from build123d import *

# Parameters (mm, degrees)
F0_R     = 1.625
F0_R_2   = 4
F0_R_3   = 3
F1_DEPTH = 4
F3_DEPTH = 25
F5_DEPTH = 2
F6_R     = 1


with BuildPart() as f1:
    # F0 (on Top) → F1 (new body)
    with BuildSketch(Plane.XY):
        with BuildLine():
            ThreePointArc((-9.4837298081, 16.9083510106), (-10.0814206469, 18.2972590095), (-11.0073593129, 19.4926406871))
            Line((-11.0073593129, 19.4926406871), (-39.7406588467, 48.2259402209))
            ThreePointArc((-39.7406588467, 48.2259402209), (-45.1494727757, 55.6091692733), (-48.0804471902, 64.2796207229))
            ThreePointArc((-48.0804471902, 64.2796207229), (-52.3618521384, 72.1460862496), (-60.5351583135, 75.8078855862))
            ThreePointArc((-60.5351583135, 75.8078855862), (-65.6898975166, 76.7624502228), (-70.5997654152, 78.5997654152))
            ThreePointArc((-70.5997654152, 78.5997654152), (-77.4281925399, 77.4281925399), (-78.5997654152, 70.5997654152))
            ThreePointArc((-78.5997654152, 70.5997654152), (-76.7624502228, 65.6898975166), (-75.8078855862, 60.5351583135))
            ThreePointArc((-75.8078855862, 60.5351583135), (-72.1460862496, 52.3618521384), (-64.2796207229, 48.0804471902))
            ThreePointArc((-64.2796207229, 48.0804471902), (-55.6091692733, 45.1494727757), (-48.2259402209, 39.7406588467))
            Line((-48.2259402209, 39.7406588467), (-19.4926406871, 11.0073593129))
            ThreePointArc((-19.4926406871, 11.0073593129), (-18.2972590095, 10.0814206469), (-16.9083510106, 9.4837298081))
            ThreePointArc((-16.9083510106, 9.4837298081), (-14.5935043457, 8.4875784101), (-12.6012015497, 6.9443473002))
            Line((-12.6012015497, 6.9443473002), (-5.6568542495, 0))
            Line((-5.6568542495, 0), (0, 0))
            Line((0, 0), (0, 5.6568542495))
            Line((0, 5.6568542495), (-6.9443473002, 12.6012015497))
            ThreePointArc((-6.9443473002, 12.6012015497), (-8.4875784101, 14.5935043457), (-9.4837298081, 16.9083510106))
        make_face()
        with Locations((-15.25, 15.25)):
            Circle(F0_R, mode=Mode.SUBTRACT)
        with Locations((-21, 21)):
            Circle(F0_R, mode=Mode.SUBTRACT)
        with Locations((-61.8718433538, 61.8718433538)):
            Circle(F0_R_2, mode=Mode.SUBTRACT)
        with Locations((-73.1855518528, 73.1855518528)):
            Circle(F0_R_3, mode=Mode.SUBTRACT)
    extrude(amount=F1_DEPTH)

    # F2 (on face) → F3 (cut)
    with BuildSketch(Plane.XY.offset(4)):
        with BuildLine():
            ThreePointArc((-55.3718433538, 63.4718433538), (-56.9718433538, 61.8718433538), (-55.3718433538, 60.2718433538))
            Line((-55.3718433538, 60.2718433538), (-52.3718433538, 60.2718433538))
            ThreePointArc((-52.3718433538, 60.2718433538), (-50.7718433538, 61.8718433538), (-52.3718433538, 63.4718433538))
            Line((-52.3718433538, 63.4718433538), (-55.3718433538, 63.4718433538))
        make_face()
        with BuildLine():
            Line((-63.4718433538, 71.3718433538), (-63.4718433538, 68.3718433538))
            ThreePointArc((-63.4718433538, 68.3718433538), (-61.8718433538, 66.7718433538), (-60.2718433538, 68.3718433538))
            Line((-60.2718433538, 68.3718433538), (-60.2718433538, 71.3718433538))
            ThreePointArc((-60.2718433538, 71.3718433538), (-61.8718433538, 72.9718433538), (-63.4718433538, 71.3718433538))
        make_face()
        with BuildLine():
            Line((-71.3718433538, 60.2718433538), (-68.3718433538, 60.2718433538))
            ThreePointArc((-68.3718433538, 60.2718433538), (-66.7718433538, 61.8718433538), (-68.3718433538, 63.4718433538))
            Line((-68.3718433538, 63.4718433538), (-71.3718433538, 63.4718433538))
            ThreePointArc((-71.3718433538, 63.4718433538), (-72.9718433538, 61.8718433538), (-71.3718433538, 60.2718433538))
        make_face()
        with BuildLine():
            Line((-60.2718433538, 52.3718433538), (-60.2718433538, 55.3718433538))
            ThreePointArc((-60.2718433538, 55.3718433538), (-61.8718433538, 56.9718433538), (-63.4718433538, 55.3718433538))
            Line((-63.4718433538, 55.3718433538), (-63.4718433538, 52.3718433538))
            ThreePointArc((-63.4718433538, 52.3718433538), (-61.8718433538, 50.7718433538), (-60.2718433538, 52.3718433538))
        make_face()
    extrude(amount=-F3_DEPTH, mode=Mode.SUBTRACT)

    # F4 (on face) → F5 (cut)
    with BuildSketch(Plane(origin=(0, 0, 0), x_dir=(1, 0, 0), z_dir=(0, 0, -1))):
        with BuildLine():
            Line((0, 0), (-20, 0))
            Line((-20, 0), (-20, -10.25))
            Line((-20, -10.25), (-15.25, -10.25))
            ThreePointArc((-15.25, -10.25), (-11.7144660941, -11.7144660941), (-10.25, -15.25))
            Line((-10.25, -15.25), (-10.25, -20))
            Line((-10.25, -20), (0, -20))
            Line((0, -20), (0, 0))
        make_face()
    extrude(amount=-F5_DEPTH, mode=Mode.SUBTRACT)

    # F6
    f6_edges = [f1.edges().sort_by_distance(p)[0] for p in [
        (0, 0, 3),
    ]]
    fillet(f6_edges, radius=F6_R)


solid = f1.part
Read the model definition and answer for the solid it produces. Units are mm, in the model's axes. A direction names the side the tool comes from. Coordinates: 2 decimals unless noted, no trailing zeros. Order: outer loops, then holes, each group sorted by start corner. A loop starts at its lowest first (then second) coordinate and runs counter-clockwise, first axis right, second up. Notation, with made-up numbers: M -35.75,-21.5 L -12.75,-21.5 A8 ccw -12.75,-15.5 Z; hole C 85,-2 d6. An arc over 180 degrees is marked long. Put each result on its own line as item: value. Start each with the question number.
Item 1: Section A-A, the plane x = -54 is taken. Determine the outline of the cut face in (y, z), plus the area to 3 significant figures.
Item 2: Given pin 1 Ø1.5 at (x, z) = (-54, 2.5) entering from +Y; pin 2 Ø1.5 at (y, z) = (54.5, 2.5) entering from +X; pin 3 Ø1.5 at (x, z) = (-70, 2) entering from +Y, each flat-ended and moving along its own axis, determine where each tip first touches the part or whether it passes through.
Item 3: The mould has two halves that part along X. Classify faces 1 (the face through (-9.178, 3.521, 2.986)), 2 (the face through (-45.09, 55.495, 1.972)), 3 (the face through (-54, 63.472, 2)): +X half, -X half, draft (parallel to the pull), parting line (faces both ways), or undercut.
Item 4: Section C-C, the plane y = 34 is taken. Determine the outline of the cut face in (x, z).
Item 5: For faces 4 (the face through (-10.249, 18.565, 2.416)), 5 (the face through (-10.25, 17, 1)), 6 (the face through (-72.97, 61.91, 2.03)), determine the directions among +Z, -Z, +X, -X, +Y, -Y from which every point of the face is accessible in a straight line to the end or side of a thin tool.
Item 6: Consider probe 1 along X at (y, z) = (71, 2.15); probe 2 along Y at (x, z) = (-62, 3.4); probe 3 along Z at (x, y) = (-9, 7). Determine where each line is inside the solid, lowest interval first. Write a range as [from, to].
Item 7: Section B-B, the plane y = 21 is taken. Determine the outline of the cut face in (x, z) (3 decimals), plus the area to 3 significant figures.
Computed:
1. outline: M 44.25,0 L 60.27,0 L 60.27,4 L 44.25,4 Z; M 63.47,0 L 73.45,0 L 73.45,4 L 63.47,4 Z
1. area: 104 mm2
2. pin 1: stops at y = 73.93
2. pin 2: stops at x = -44.1
2. pin 3: stops at y = 78.67
3. face 1: -X half
3. face 2: +X half
3. face 3: undercut
4. outline: M -42.49,0 L -25.51,0 L -25.51,4 L -42.49,4 Z
5. face 4: +Z, -Z, +X, +Y
5. face 5: -Z, +X, +Y, -Y
5. face 6: +Z, -Z
6. probe 1: x = [-78.77, -75.24], [-71.13, -63.47], [-60.27, -51.26]
6. probe 2: y = [47.59, 50.78], [56.97, 57.87], [65.87, 66.78], [72.97, 75.98]
6. probe 3: z = [2, 4]
7. outline: M -29.485,0 L -22.625,0 L -22.625,4 L -29.485,4 Z; M -19.375,0 L -12.515,0 L -12.515,4 L -19.375,4 Z
7. area: 54.9 mm2
